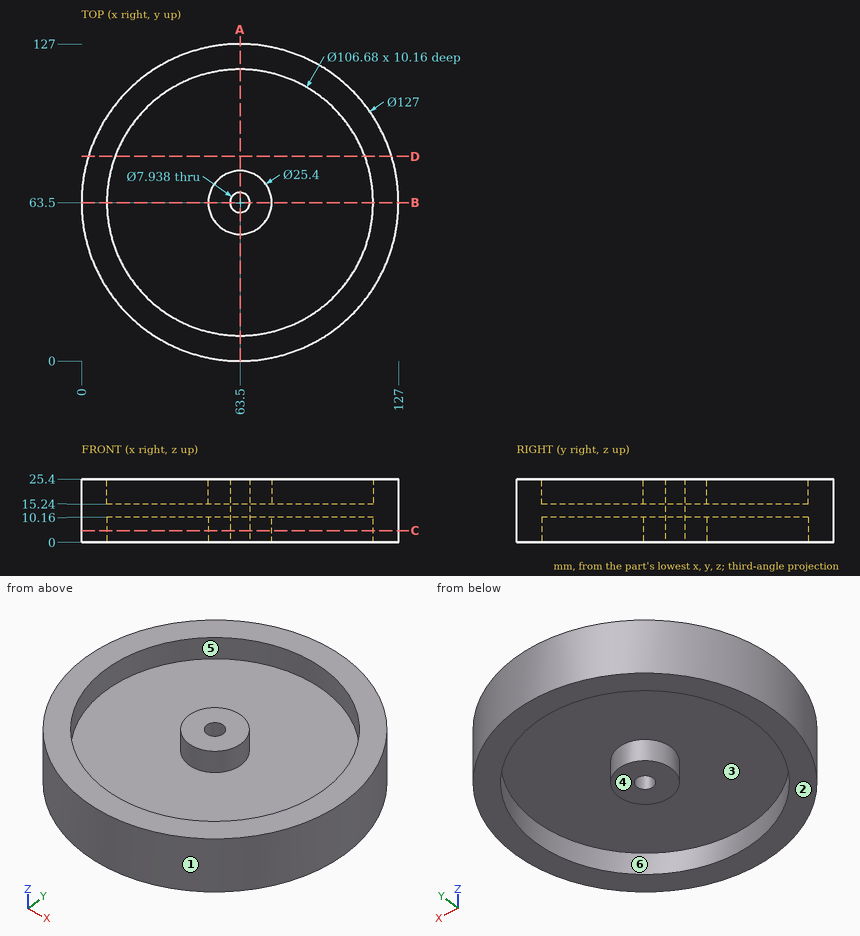
Job drawing, mm, ordinate dimensions from the low corner. One solid piece. A direction names the side the tool comes from. Coordinates: 2 decimals unless noted, no trailing zeros. Loops run counter-clockwise (first coordinate to the right, second up) from the corner with the lowest first, then second, coordinate; pieces in that order, holes last. Notation, with made-up numbers: (81, 35.25) - (96, 35.25) arc R15 ccw to (96, 53.25) - close; hole circle Ø7 at (3.25, -4.5). An arc over 180 degrees is marked (long way). Write item = value, one per line. Start each with the question number.
Q1. Flat gauge pins, fed straight in: pin 1 Ø12 at (y, z) = (82, 23) entering from +X; pin 2 Ø1.5 at (x, z) = (92, 22) entering from -Y (1 decimal); pin 3 Ø12 at (x, z) = (50.5, 17.5) entering from -Y; pin 4 Ø10.5 at (x, y) = (63.5, 63.5) entering from +Z. Where does each tip first touch, or does it go through?
Q2. Cut at A-A, the plane x = 63.5. List the corners of the cut face in (y, z), then the cut area to 3 significant figures.
Q3. Cut at D-D, the plane y = 82. List the corners of the cut face in (x, z) (1 decimal), then the cut area to 3 significant figures.
Q4. Pull direction X, two halves, no side cores. Call the marked faces 1, 2 and 3: pulls with the +X half, pulls with the -X half, needs draft (parallel to the pull), parting line crosses it, or undercut.
Q5. Which spindle directions (+Z, -Z, +X, -X, +Y, -Y) get a long thin tool onto all of the face, cutting with end or side? Do the marked faces 4, 5 and 6. Say none if no direction does.
Q6. Cut at C-C, the plane z = 4.75. List the corners of the cut face in (x, y), then the cut area to 3 significant figures.
Q7. Drill centre lines: L1, parallel to Y at x = 63.5, z = 8.25; L2, parallel to Z at x = 40, y = 87.5; L3, parallel to Y at x = 58, z = 18 (1 decimal). Where is each one in solid material? Low to high.
Computed:
q1.pin_1 = 125.76
q1.pin_2 = 6.4
q1.pin_3 = 0.39
q1.pin_4 = 25.4
q2.outline = (0, 0) - (10.16, 0) - (10.16, 10.16) - (50.8, 10.16) - (50.8, 0) - (59.53, 0) - (59.53, 25.4) - (50.8, 25.4) - (50.8, 15.24) - (10.16, 15.24) - (10.16, 25.4) - (0, 25.4) - close; (67.47, 0) - (76.2, 0) - (76.2, 10.16) - (116.84, 10.16) - (116.84, 0) - (127, 0) - (127, 25.4) - (116.84, 25.4) - (116.84, 15.24) - (76.2, 15.24) - (76.2, 25.4) - (67.47, 25.4) - close
q2.area = 1,370 mm²
q3.outline = (2.8, 0) - (13.5, 0) - (13.5, 10.2) - (113.5, 10.2) - (113.5, 0) - (124.2, 0) - (124.2, 25.4) - (113.5, 25.4) - (113.5, 15.2) - (13.5, 15.2) - (13.5, 25.4) - (2.8, 25.4) - close
q3.area = 1,050 mm²
q4.face_1 = parting line crosses it
q4.face_2 = needs draft
q4.face_3 = undercut
q5.face_4 = -Z, +X, -X, +Y, -Y
q5.face_5 = +Z
q5.face_6 = -Z
q6.outline = circle Ø127 at (63.5, 63.5); circle Ø25.4 at (63.5, 63.5); hole circle Ø106.68 at (63.5, 63.5); hole circle Ø7.94 at (63.5, 63.5)
q6.area = 4,190 mm²
q7.L1 = 0 to 10.16, 50.8 to 59.53, 67.47 to 76.2, 116.84 to 127
q7.L2 = 10.16 to 15.24
q7.L3 = 0.2 to 10.4, 52.1 to 74.9, 116.6 to 126.8
